```python
from build123d import *

# Parameters (mm, degrees)
ESBO_O1_R                = 10
RESSALTO_EXTRUS_O1_DEPTH = 15
ESBO_O2_W                = 10
ESBO_O2_H                = 36.681278326
CORTE_EXTRUS_O1_DEPTH    = 41


with BuildPart() as part:
    # Esboço1 → Ressalto-extrusão1 (new body, symmetric)
    with BuildSketch(Plane.XY):
        with BuildLine():
            Line((-20, 0), (20, 0))
            Line((20, 0), (20, 20))
            ThreePointArc((20, 20), (0, 40), (-20, 20))
            Line((-20, 20), (-20, 0))
        make_face()
        with Locations((0, 20)):
            Circle(ESBO_O1_R, mode=Mode.SUBTRACT)
    extrude(amount=RESSALTO_EXTRUS_O1_DEPTH, both=True)

    # Esboço2 → Corte-extrusão1 (cut, through all)
    with BuildSketch(Plane(origin=(20, 0, 0), x_dir=(0, 0, -1), z_dir=(1, 0, 0))):
        with Locations((0, 28.340639163)):
            Rectangle(ESBO_O2_W, ESBO_O2_H)
    extrude(amount=-CORTE_EXTRUS_O1_DEPTH, mode=Mode.SUBTRACT)


solid = part.part
```
Check sheet for the modelled part. Datum: model origin and axes. Units: mm. A direction names the side the tool comes from. Give positions to 0.01 mm unless a question says otherwise; leave off trailing zeros. Write each loop counter-clockwise with the first axis right and the second up, starting at its lowest first coordinate (ties: lowest second). Pieces come first, ordered by that corner, then holes.
Item 1: Draft check along Z on faces 1 (the face through (0, 10, 0)), 2 (the face through (0, 7, -15)), 3 (the face through (0, 7, 15)). Enter one of: released by +Z, released by -Z, zero draft, split by the parting line, or undercut.
Item 2: Cross-section at A-A (y = 12). Enter the section's corners in (x, z), and give its area (3 significant figures).
Item 3: Access from +Z, -Z, +X, -X, +Y, -Y to the whole of each face (thin tool, end or side, straight path). Record for faces 4 (the face through (0, 31, -5)), 5 (the face through (20, 8, 0)).
Item 4: Cross-section at B-B (y = 36). Enter the section's corners in (x, z), and give its area (3 significant figures).
Item 5: Cross-section at C-C (x = 7). Enter the section's corners in (y, z) (3 decimals).
Item 6: Gauge pin test, flat ends, axial feed: pin 1 (12 mm diameter, centred on x = 0, y = 20, fed in from -Z); pin 2 (4 mm diameter, centred on x = 3, z = -9.5, fed in from +Y) (3 decimals); pin 3 (6 mm diameter, centred on x = -10, z = -10, fed in from +Y) (3 decimals); pin 4 (2 mm diameter, centred on x = -4, z = 1.5, fed in from +Y). Record the tip position at first contact, or that the pin passes through.
Item 7: Scan lines: L1, parallel to X at y = 20, z = 8.25; L2, parallel to Z at x = 10, y = 22; L3, parallel to Y at x = 0, z = 13. Record each from-to range of solid material in increasing order.
Item 8: Cross-section at D-D (z = 12.5). Enter the section's corners in (x, y).
Report:
1. face 1: undercut
1. face 2: released by -Z
1. face 3: released by +Z
2. outline: (-20, -15) - (-6, -15) - (-6, -5) - (-20, -5) - close; (-20, 5) - (-6, 5) - (-6, 15) - (-20, 15) - close; (6, -15) - (20, -15) - (20, -5) - (6, -5) - close; (6, 5) - (20, 5) - (20, 15) - (6, 15) - close
2. area: 560 mm2
3. face 4: +X, -X, +Y
3. face 5: +Z, -Z, +X, +Y, -Y
4. outline: (-12, -15) - (12, -15) - (12, -5) - (-12, -5) - close; (-12, 5) - (12, 5) - (12, 15) - (-12, 15) - close
4. area: 480 mm2
5. outline: (0, -15) - (12.859, -15) - (12.859, -5) - (10, -5) - (10, 5) - (12.859, 5) - (12.859, 15) - (0, 15) - close; (27.141, -15) - (38.735, -15) - (38.735, -5) - (27.141, -5) - close; (27.141, 5) - (38.735, 5) - (38.735, 15) - (27.141, 15) - close
6. pin 1: passes through
6. pin 2: stops at y = 39.975
6. pin 3: stops at y = 38.735
6. pin 4: stops at y = 10
7. L1: x = -20 to -10, 10 to 20
7. L2: z = -15 to -5, 5 to 15
7. L3: y = 0 to 10, 30 to 40
8. outline: (-20, 0) - (20, 0) - (20, 20) arc R20 ccw to (-20, 20) - close; hole circle Ø20 at (0, 20)
